from build123d import *

# Parameters (mm, degrees)
EXTRUDE_1_DEPTH = 3
CHAMFER_1_SIZE  = 0.5


with BuildPart() as part:
    # 草图1 → 凸台-拉伸1 (new body)
    with BuildSketch(Plane.XY):
        Polygon((84.803847577, -9), (-93.196152423, -9), (-94.196152423, -7.267949192), (-84.803847577, 9), (93.196152423, 9), (94.196152423, 7.267949192), align=None)
    extrude(amount=EXTRUDE_1_DEPTH)

    # 倒角1
    chamfer_1_edges = [part.edges().sort_by_distance(p)[0] for p in [
        (4.196152423, 9, 3),
        (-89.5, 0.866025404, 3),
        (-93.696152423, -8.133974596, 3),
        (-4.196152423, -9, 3),
        (89.5, -0.866025404, 3),
        (-4.196152423, -9, 0),
        (-93.696152423, -8.133974596, 0),
        (-89.5, 0.866025404, 0),
        (4.196152423, 9, 0),
        (93.696152423, 8.133974596, 0),
        (89.5, -0.866025404, 0),
        (93.696152423, 8.133974596, 3),
    ]]
    chamfer(chamfer_1_edges, length=CHAMFER_1_SIZE)


solid = part.part
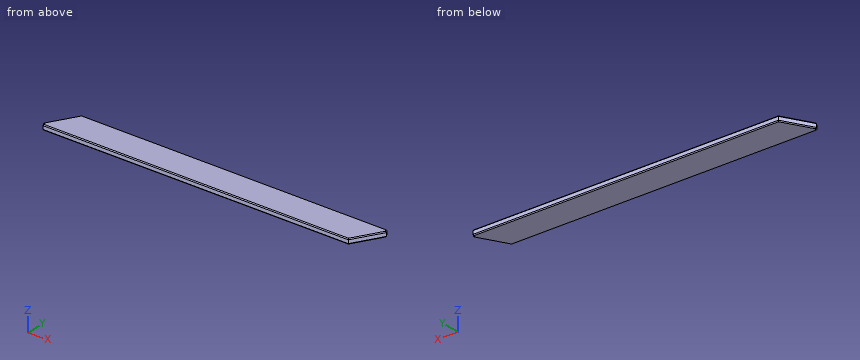
Geometry: final body of the model. Coordinates: model frame, mm. Coordinates: 2 decimals unless noted, no trailing zeros. Order: outer loops, then holes, each group sorted by start corner. A loop starts at its lowest first (then second) coordinate and runs counter-clockwise, first axis right, second up. Notation, with made-up numbers: M 4,20.5 L 38,20.5 A26 cw 38,44.5 Z; hole C -33,14 d9. An arc over 180 degrees is marked long. One line per question, with ' | ' between items. Start each with the question number.
Item 1: Cut plane A-A, the plane y = 2.5. Return the cut outline in (x, z), then the cut area to 3 significant figures.
Item 2: Ray query, probe 1 along X at (y, z) = (-1.75, 1.8); probe 2 along X at (y, z) = (-7.75, 1.35); probe 3 along Y at (x, z) = (-69.5, 2.85). Return the intervals inside material, ascending. Write a range as [from, to].
Item 3: Pin query (flat end, axial travel): pin 1 Ø1 at (y, z) = (1.5, 2.5) entering from +X. Return the tip coordinate at first contact, or that it passes through.
Item 4: Cut plane B-B, the plane z = 1.05. Return the cut outline in (x, y), then the cut area to 3 significant figures.
A:
1) outline: M -88.56,0.5 L -87.98,0 L 90.87,0 L 91.44,0.5 L 91.44,2.5 L 90.87,3 L -87.98,3 L -88.56,2.5 Z | area: 539 mm2
2) probe 1: x = [-91.01, 88.99] | probe 2: x = [-93.92, 85.53] | probe 3: y = [-8.65, 8.65]
3) pin 1: stops at x = 91.15
4) outline: M -94.2,-7.27 L -93.2,-9 L 84.8,-9 L 94.2,7.27 L 93.2,9 L -84.8,9 Z | area: 3,240 mm2
